Here's how the part is built. I have some questions about the finished solid (model axes, mm). Face numbers are marked on the shaded views. A direction names the side the tool comes from. Round coordinates to 2 decimals unless told otherwise and drop trailing zeros. Loops run counter-clockwise (first coordinate to the right, second up) from the corner with the lowest first, then second, coordinate; pieces in that order, holes last. Notation, with made-up numbers: M 15.5,35.5 L 20.5,35.5 A12 cw 20.5,53.5 Z; hole C 66.25,14.25 d6. An arc over 180 degrees is marked long. Answer as CSV lines item,"result".
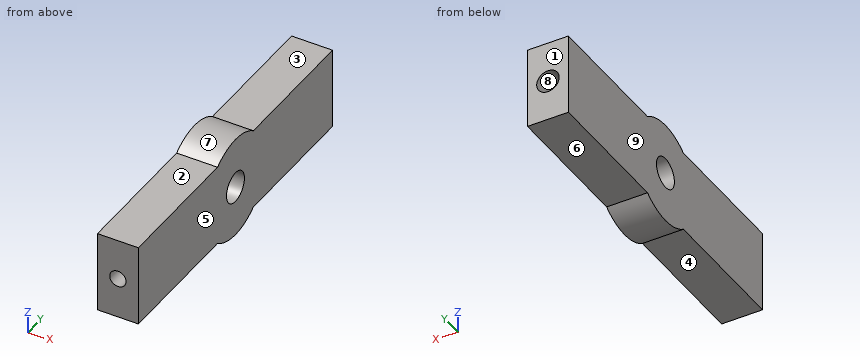
Autodesk Inventor part; units mm, degrees
ref_plane "YZ Plane" through (0, 0, 0) normal (1, 0, 0) x (0, 1, 0)
ref_plane "XZ Plane" through (0, 0, 0) normal (0, 1, 0) x (-1, 0, 0)
ref_plane "XY Plane" through (0, 0, 0) normal (0, 0, 1) x (1, 0, 0)
sketch "スケッチ1" plane through (0, 0, 0) normal (0, 1, 0) x (-1, 0, 0)
  line L0 (-2, 4) -> (2, 4)
  line L1 (2, 4) -> (2, -4)
  line L2 (2, -4) -> (-2, -4)
  line L3 (-2, -4) -> (-2, 4)
  line L4 (-2, 4) -> (2, -4) construction
  line L5 (2, 4) -> (-2, -4) construction
  circle A0 centre (0, 0) radius 1
  dimension "d0" = 8
  dimension "d1" = 4
  dimension "d2" = 2
extrude "押し出し1" add sketch "スケッチ1" along normal blind 32.5 contours L0 L1 L2 L3 | A0
sketch "スケッチ2" plane through (0, 0, 0) normal (0, -1, 0) x (1, 0, 0)
  circle A0 centre (0, 0) radius 0.8
  dimension "d5" = 1.6
extrude "押し出し2" cut sketch "スケッチ2" against normal blind 6
sketch "スケッチ3" plane through (2, 0, 4) normal (1, 0, 0) x (0, 0, -1)
  circle A0 centre (4, 24.25) radius 1.5 construction
  circle A1 centre (4, 8.25) radius 1.5 construction
  line L0 (8, 32.5) -> (0, 32.5)
  line L1 (4, 32.5) -> (4, 0)
  line L2 (4, 0) -> (3.3318, 0)
  line L3 (4, 32.5) -> (4, 24.25) construction
  line L4 (4, 24.25) -> (4, 8.25) construction
  line L5 (4, 8.25) -> (4, 0) construction
  line L6 (0, 0) -> (8, 0)
  line L7 (0, 32.5) -> (8, 32.5)
  circle A2 centre (4, 16.25) radius 1.5
  dimension "d8" = 3
  dimension "d9" = 16
  dimension "d15" = 3
extrude "押し出し3" cut sketch "スケッチ3" against normal up to surface (4 mm away)
sketch "スケッチ4" plane through (0, 32.5, 0) normal (0, 1, 0) x (1, 0, 0)
  circle A0 centre (0, 0) radius 1.1
  dimension "d12" = 2.2
extrude "押し出し4" cut sketch "スケッチ4" against normal blind 6
sketch "スケッチ5" plane through (2, 0, 4) normal (1, 0, 0) x (0, 0, -1)
  circle A0 centre (4, 16.25) radius 1.5
  line L0 (0, 0) -> (8, 0)
  line L1 (8, 0) -> (8, 32.5)
  line L2 (0, 32.5) -> (8, 32.5)
  line L3 (0, 0) -> (0, 32.5)
  circle A1 centre (4, 16.25) radius 5
  point P0 (4, 0)
  dimension "d16" = 10
extrude "押し出し5" add sketch "スケッチ5" against normal up to surface (4 mm away) contours A1 L3 | L3 A1 L1 | L1 A1
properties part number "BallSensor"
1. If I drill on line 1 (Y direction, x = 1, z = 0); line 2 (Y direction, x = 0.3, z = 0); line 3 (Z direction, x = 0.8, y = 16.25), over which ranges is the centre line in solid material (lowest first)? Write a range as [from, to].
Evaluation:
line 1,"y = [0, 14.75], [17.75, 26.5]"
line 2,"y = [6, 14.75], [17.75, 26.5]"
line 3,"z = [-5, -1.5], [1.5, 5]"
2. I want a section at C-C, the plane x = 0. Please give me the cut outline in (y, z), and give its area (3 significant figures).
Evaluation:
outline,"M 0,-4 L 13.25,-4 A5 ccw 19.25,-4 L 32.5,-4 L 32.5,-1.1 L 26.5,-1.1 L 26.5,1.1 L 32.5,1.1 L 32.5,4 L 19.25,4 A5 ccw 13.25,4 L 0,4 L 0,0.8 L 6,0.8 L 6,-0.8 L 0,-0.8 Z; hole C 16.25,0 d3"
area,"238 mm²"
3. I want a section at D-D, the plane x = -1.6. Please give me the cut outline in (y, z).
Evaluation:
outline,"M 0,-4 L 13.25,-4 A5 ccw 19.25,-4 L 32.5,-4 L 32.5,4 L 19.25,4 A5 ccw 13.25,4 L 0,4 Z; hole C 16.25,0 d3"
4. Which directions (+Z, -Z, +X, -X, +Y, -Y) give clear straight access to the entire face, cutting with the end or side of a thin tool? Please do the marked faces 1, 2, 3, 4 and 5.
Evaluation:
face 1,"+Z, -Z, +X, -X, +Y"
face 2,"+Z, +X, -X, -Y"
face 3,"+Z, +X, -X, +Y"
face 4,"-Z, +X, -X, -Y"
face 5,"+Z, -Z, +X, +Y, -Y"
5. For P1, Ø0.7, axis at x = -0.5, z = 0, coming from the +Y side; P2, Ø2, axis at x = -1, y = 25.5, coming from the -Z side; P3, Ø1.2, axis at x = 1, y = 7, coming from the +Z side, each with a flat end and sliding along its axis, tell me the tip position at first contact or that it passes through.
Evaluation:
P1,"stops at y = 26.5"
P2,"stops at z = -4"
P3,"stops at z = 4"
6. We'd pull the mould along Z, two halves only. Please class the marked faces 6, 7, 8 and 9: pulls with the +Z half, pulls with the -Z half, needs draft (parallel to the pull), parting line crosses it, or undercut.
Evaluation:
face 6,"pulls with the -Z half"
face 7,"pulls with the +Z half"
face 8,"undercut"
face 9,"needs draft"
7. I want a section at A-A, the plane y = 16.25. Please give me the cut outline in (x, z), and give its area (3 significant figures).
Evaluation:
outline,"M -2,-5 L 2,-5 L 2,-1.5 L -2,-1.5 Z; M -2,1.5 L 2,1.5 L 2,5 L -2,5 Z"
area,"28.0 mm²"
8. I want a section at B-B, the plane z = 0. Please give me the cut outline in (x, y).
Evaluation:
outline,"M -2,0 L -0.8,0 L -0.8,6 L 0.8,6 L 0.8,0 L 2,0 L 2,14.75 L -2,14.75 Z; M -2,17.75 L 2,17.75 L 2,32.5 L 1.1,32.5 L 1.1,26.5 L -1.1,26.5 L -1.1,32.5 L -2,32.5 Z"
